```python
from build123d import *

# Parameters (mm, degrees)
BOSS_EXTRUDE1_DEPTH = 9.7
SKETCH5_R           = 2
BOSS_EXTRUDE2_DEPTH = 7.5
SKETCH6_R           = 7.05
BOSS_EXTRUDE3_DEPTH = 2


with BuildPart() as part:
    # Sketch1 → Boss-Extrude1 (new body)
    with BuildSketch(Plane.XY):
        with BuildLine():
            Line((-3.247465815, 9.036994825), (-1.879385242, 12.795765308))
            ThreePointArc((-1.879385242, 12.795765308), (0, 14.111725022), (1.879385242, 12.795765308))
            Line((1.879385242, 12.795765308), (3.247465815, 9.036994825))
            Line((3.247465815, 9.036994825), (6.202534185, 7.330885306))
            Line((6.202534185, 7.330885306), (10.141765197, 8.025478017))
            ThreePointArc((10.141765197, 8.025478017), (12.22111236, 7.055862511), (12.021150439, 4.770287292))
            Line((12.021150439, 4.770287292), (9.45, 1.706109519))
            Line((9.45, 1.706109519), (9.45, -1.706109519))
            Line((9.45, -1.706109519), (12.021150439, -4.770287292))
            ThreePointArc((12.021150439, -4.770287292), (12.22111236, -7.055862511), (10.141765197, -8.025478017))
            Line((10.141765197, -8.025478017), (6.202534185, -7.330885306))
            Line((6.202534185, -7.330885306), (3.247465815, -9.036994825))
            Line((3.247465815, -9.036994825), (1.879385242, -12.795765308))
            ThreePointArc((1.879385242, -12.795765308), (0, -14.111725022), (-1.879385242, -12.795765308))
            Line((-1.879385242, -12.795765308), (-3.247465815, -9.036994825))
            Line((-3.247465815, -9.036994825), (-6.202534185, -7.330885306))
            Line((-6.202534185, -7.330885306), (-10.141765197, -8.025478017))
            ThreePointArc((-10.141765197, -8.025478017), (-12.22111236, -7.055862511), (-12.021150439, -4.770287292))
            Line((-12.021150439, -4.770287292), (-9.45, -1.706109519))
            Line((-9.45, -1.706109519), (-9.45, 1.706109519))
            Line((-9.45, 1.706109519), (-12.021150439, 4.770287292))
            ThreePointArc((-12.021150439, 4.770287292), (-12.22111236, 7.055862511), (-10.141765197, 8.025478017))
            Line((-10.141765197, 8.025478017), (-6.202534185, 7.330885306))
            Line((-6.202534185, 7.330885306), (-3.247465815, 9.036994825))
        make_face()
        Polygon((3.45, -1.991858429), (3.45, 1.991858429), (0, 3.983716857), (-3.45, 1.991858429), (-3.45, -1.991858429), (0, -3.983716857), align=None, mode=Mode.SUBTRACT)
    extrude(amount=BOSS_EXTRUDE1_DEPTH)

    # Sketch5 → Boss-Extrude2 (add)
    with BuildSketch(Plane(origin=(0, 0, 0), x_dir=(-1, 0, 0), z_dir=(0, 0, -1))):
        Polygon((-3.45, 1.991858429), (0, 3.983716857), (3.45, 1.991858429), (3.45, -1.991858429), (0, -3.983716857), (-3.45, -1.991858429), align=None)
        Circle(SKETCH5_R, mode=Mode.SUBTRACT)
    extrude(amount=-BOSS_EXTRUDE2_DEPTH)

    # Sketch6 → Boss-Extrude3 (add)
    with BuildSketch(Plane.XY.offset(9.7)):
        with BuildLine():
            Line((-3.247465815, 9.036994825), (-6.202534185, 7.330885306))
            Line((-6.202534185, 7.330885306), (-10.141765197, 8.025478017))
            ThreePointArc((-10.141765197, 8.025478017), (-12.22111236, 7.055862511), (-12.021150439, 4.770287292))
            Line((-12.021150439, 4.770287292), (-9.45, 1.706109519))
            Line((-9.45, 1.706109519), (-9.45, -1.706109519))
            Line((-9.45, -1.706109519), (-12.021150439, -4.770287292))
            ThreePointArc((-12.021150439, -4.770287292), (-12.22111236, -7.055862511), (-10.141765197, -8.025478017))
            Line((-10.141765197, -8.025478017), (-6.202534185, -7.330885306))
            Line((-6.202534185, -7.330885306), (-3.247465815, -9.036994825))
            Line((-3.247465815, -9.036994825), (-1.879385242, -12.795765308))
            ThreePointArc((-1.879385242, -12.795765308), (0, -14.111725022), (1.879385242, -12.795765308))
            Line((1.879385242, -12.795765308), (3.247465815, -9.036994825))
            Line((3.247465815, -9.036994825), (6.202534185, -7.330885306))
            Line((6.202534185, -7.330885306), (10.141765197, -8.025478017))
            ThreePointArc((10.141765197, -8.025478017), (12.22111236, -7.055862511), (12.021150439, -4.770287292))
            Line((12.021150439, -4.770287292), (9.45, -1.706109519))
            Line((9.45, -1.706109519), (9.45, 1.706109519))
            Line((9.45, 1.706109519), (12.021150439, 4.770287292))
            ThreePointArc((12.021150439, 4.770287292), (12.22111236, 7.055862511), (10.141765197, 8.025478017))
            Line((10.141765197, 8.025478017), (6.202534185, 7.330885306))
            Line((6.202534185, 7.330885306), (3.247465815, 9.036994825))
            Line((3.247465815, 9.036994825), (1.879385242, 12.795765308))
            ThreePointArc((1.879385242, 12.795765308), (0, 14.111725022), (-1.879385242, 12.795765308))
            Line((-1.879385242, 12.795765308), (-3.247465815, 9.036994825))
        make_face()
        Circle(SKETCH6_R, mode=Mode.SUBTRACT)
    extrude(amount=BOSS_EXTRUDE3_DEPTH)


solid = part.part
```
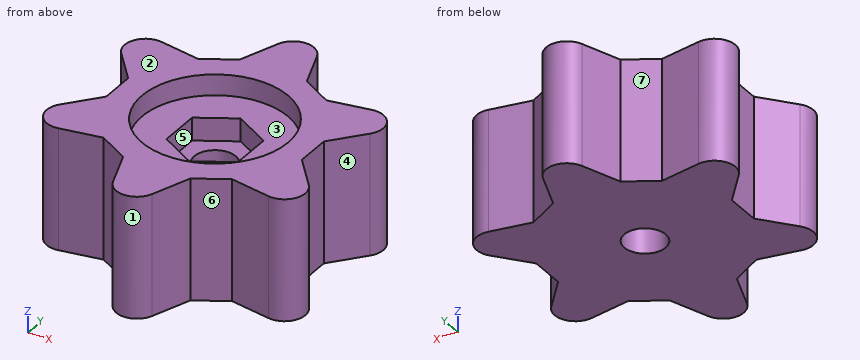
The model under review builds one solid part; all positions refer to its coordinate system, in mm. Face numbers are marked on the shaded views. A direction names the side the tool comes from. Round coordinates to 2 decimals unless told otherwise and drop trailing zeros. Loops run counter-clockwise (first coordinate to the right, second up) from the corner with the lowest first, then second, coordinate; pieces in that order, holes last.
1) Consider section A-A on z = 2. State the section outline as (x, y) points.
Values follow:
outline: (-12.02, -4.77) arc R2 ccw to (-10.14, -8.03) - (-6.2, -7.33) - (-3.25, -9.04) - (-1.88, -12.8) arc R2 ccw to (1.88, -12.8) - (3.25, -9.04) - (6.2, -7.33) - (10.14, -8.03) arc R2 ccw to (12.02, -4.77) - (9.45, -1.71) - (9.45, 1.71) - (12.02, 4.77) arc R2 ccw to (10.14, 8.03) - (6.2, 7.33) - (3.25, 9.04) - (1.88, 12.8) arc R2 ccw to (-1.88, 12.8) - (-3.25, 9.04) - (-6.2, 7.33) - (-10.14, 8.03) arc R2 ccw to (-12.02, 4.77) - (-9.45, 1.71) - (-9.45, -1.71) - close; hole circle Ø4 at (0, 0)
2) Consider section B-B on y = 0. State the section outline as (x, z) points.
Values follow:
outline: (-9.45, 0) - (-2, 0) - (-2, 7.5) - (-3.45, 7.5) - (-3.45, 9.7) - (-7.05, 9.7) - (-7.05, 11.7) - (-9.45, 11.7) - close; (2, 0) - (9.45, 0) - (9.45, 11.7) - (7.05, 11.7) - (7.05, 9.7) - (3.45, 9.7) - (3.45, 7.5) - (2, 7.5) - close
3) Consider section C-C on x = 0.5. State the section outline as (y, z) points.
Values follow:
outline: (-14.05, 0) - (-1.94, 0) - (-1.94, 7.5) - (-3.7, 7.5) - (-3.7, 9.7) - (-7.03, 9.7) - (-7.03, 11.7) - (-14.05, 11.7) - close; (1.94, 0) - (14.05, 0) - (14.05, 11.7) - (7.03, 11.7) - (7.03, 9.7) - (3.7, 9.7) - (3.7, 7.5) - (1.94, 7.5) - close
4) Consider section D-D on y = -3.25. State the section outline as (x, z) points.
Values follow:
outline: (-10.75, 0) - (10.75, 0) - (10.75, 11.7) - (6.26, 11.7) - (6.26, 9.7) - (1.27, 9.7) - (1.27, 7.5) - (-1.27, 7.5) - (-1.27, 9.7) - (-6.26, 9.7) - (-6.26, 11.7) - (-10.75, 11.7) - close
5) Wall thickness on line 1 along Y through (x, z) = (0, 5.5); line 2 along Z through (x, y) = (4.5, 1.5); line 3 along Y through (x, z) = (-5, 7.5): over which ranges is each line inside the solid? List them lowest first.
Values follow:
line 1: y = -14.11 to -2, 2 to 14.11
line 2: z = 0 to 9.7
line 3: y = -8.03 to 8.03
6) The part is to be moulded in two halves that separate along X. For the marked faces 1, 2, 3 and 4, say which applies: pulls with the +X half, pulls with the -X half, needs draft (parallel to the pull), parting line crosses it, or undercut.
Values follow:
face 1: parting line crosses it
face 2: needs draft
face 3: undercut
face 4: pulls with the +X half
7) Clearance check with flat-ended pins moving along their axes: P1, Ø3, axis at x = 0, y = 0, coming from the -Z side; P2, Ø1.5, axis at x = 0, y = -2, coming from the +Z side; P3, Ø4, axis at y = -0.5, z = 4.5, coming from the -X side; P4, Ø0.7, axis at y = 0, z = 8, coming from the +X side. State where each tip first meets the part, or that it passes through.
Values follow:
P1: passes through
P2: stops at z = 7.5
P3: stops at x = -10.12
P4: stops at x = 9.45
8) Tool access review of the marked faces 5, 6 and 7: name each direction out of +Z, -Z, +X, -X, +Y, -Y from which nothing blocks a thin tool from reaching the whole face with its end or side.
Values follow:
face 5: +Z
face 6: +Z, -Z, -Y
face 7: +Z, -Z, +Y
